The figure shows three views and two pictorial views of one solid part (mm, origin at its lowest corner). Answer the questions. Give positions to 0.01 mm unless a question says otherwise; leave off trailing zeros. Order: outer loops, then holes, each group sorted by start corner. A loop starts at its lowest first (then second) coordinate and runs counter-clockwise, first axis right, second up. Notation, with made-up numbers: (-38.75, 65.25) - (-28.75, 65.25) arc R21 ccw to (-28.75, 101.25) - close; hole circle Ø6 at (2.5, -21.75). An arc over 180 degrees is marked (long way). Answer as CSV lines item,"result". Start each with the question number.
1. Flat-ended cylindrical pins translate along their axes: pin 1 (15 mm diameter, centred on x = 439, z = 215, fed in from +Y); pin 2 (6 mm diameter, centred on x = 1379.5, y = 607.5, fed in from -Z); pin 3 (15 mm diameter, centred on y = 1401.5, z = 393.5, fed in from -X). Find the tip coordinate at first contact, or state that the pin passes through.
2. Section B-B on y = 914.4 is taken. Give the vertices of the cut face in (x, z).
3. Consider line 1 along Z through (x, y) = (1091.5, 1091.5); line 2 along Y through (x, z) = (1399.5, 489.5). Determine where each line is inside the solid, lowest interval first. Write a range as [from, to].
4. Section A-A on z = 387 is taken. Give the vertices of the cut face in (x, y).
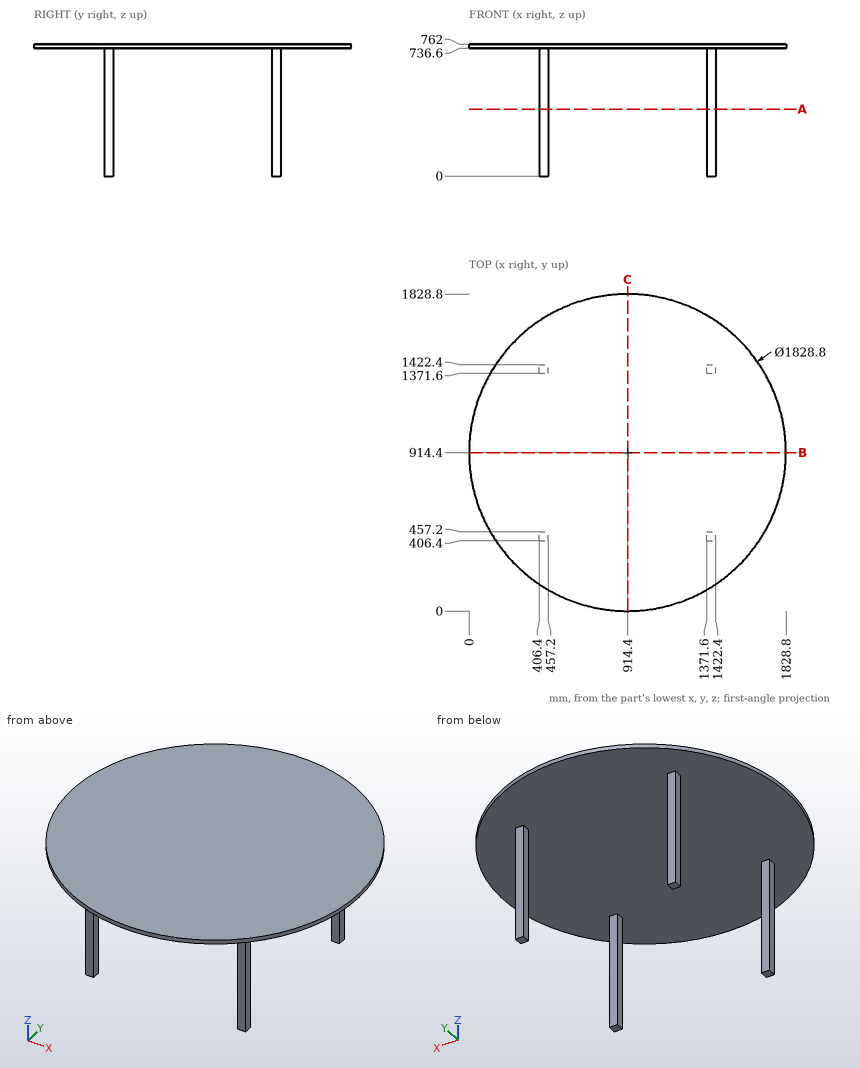
Checks:
1,pin 1,"stops at y = 1422.4"
1,pin 2,"stops at z = 736.6"
1,pin 3,"stops at x = 406.4"
2,outline,"(0, 736.6) - (1828.8, 736.6) - (1828.8, 762) - (0, 762) - close"
3,line 1,"z = [736.6, 762]"
3,line 2,"y = [406.4, 457.2], [1371.6, 1422.4]"
4,outline,"(406.4, 406.4) - (457.2, 406.4) - (457.2, 457.2) - (406.4, 457.2) - close; (406.4, 1371.6) - (457.2, 1371.6) - (457.2, 1422.4) - (406.4, 1422.4) - close; (1371.6, 406.4) - (1422.4, 406.4) - (1422.4, 457.2) - (1371.6, 457.2) - close; (1371.6, 1371.6) - (1422.4, 1371.6) - (1422.4, 1422.4) - (1371.6, 1422.4) - close"
